Check sheet for the modelled part. Datum: model origin and axes. Units: mm. A direction names the side the tool comes from. Coordinates: 2 decimals unless noted, no trailing zeros. Loops run counter-clockwise (first coordinate to the right, second up) from the corner with the lowest first, then second, coordinate; pieces in that order, holes last. Notation, with made-up numbers: (64, 70.5) -> (97, 70.5) arc R27 ccw to (97, 102.5) -> close; hole circle Ø6 at (88, 87.5). An arc over 180 degrees is marked (long way). Use CSV: the item, a comma, the result in double quotes. Start each with the question number.
1. Sectioned sample at B-B, the plane x = 4. Record the cut outline in (y, z).
2. Set-up check for faces 1 (the face through (5, 6, 9)), 2 (the face through (5, 27.395, 10)), 3 (the face through (5, 14.942, 55)), 4 (the face through (5, -6.058, 56)): record each of +Z, -Z, +X, -X, +Y, -Y from which the full face is reachable in a straight line by a thin tool's end or side.
3. Sectioned sample at D-D, the plane z = 53.5. Record the cut outline in (x, y).
4. Thickness scan on L1, parallel to Z at x = 7.75, y = 19; L2, parallel to Y at x = 4.25, z = 61; L3, parallel to Z at x = 8, y = 9. Record the ranges inside material, lowest first.
5. Release check for a two-part mould opening along Y. For faces 5 (the face through (8, 12.395, 9)), 6 (the face through (5, 21, 24)), 7 (the face through (5, -16.003, 11)) record: pulls with the +Y half, pulls with the -Y half, needs draft (parallel to the pull), parting line crosses it, or undercut.
6. Sectioned sample at C-C, the plane y = 8.5. Record the cut outline in (x, z), and give its area (3 significant figures).
7. Sectioned sample at A-A, the plane z = 6. Record the cut outline in (x, y).
8. Gauge pin test, flat ends, axial feed: pin 1 (4 mm diameter, centred on x = 8.5, y = 8.5, fed in from -Z); pin 2 (2 mm diameter, centred on x = 3.5, y = -11.5, fed in from +Z); pin 3 (5 mm diameter, centred on x = 4.5, y = -6.5, fed in from +Z). Record the tip position at first contact, or that the pin passes through.
```python
from build123d import *

# Parameters (mm, degrees)
SALIENTE_EXTRUIR1_DEPTH = 10
CROQUIS2_W              = 18
CROQUIS2_H              = 12.394708995
CORTAR_EXTRUIR1_DEPTH   = 5
REDONDEO1_R             = 3
REDONDEO2_R             = 3
REDONDEO3_R             = 1


with BuildPart() as part:
    # Croquis1 → Saliente-Extruir1 (new body)
    with BuildSketch(Plane(origin=(0, 0, 0), x_dir=(0, 0, -1), z_dir=(1, 0, 0))):
        Polygon((0, -10.216508635), (0, 27.394708995), (-24, 27.394708995), (-24, 14.942424084), (-87.663818946, 14.942424084), (-87.663818946, -6.057575916), (-24, -6.057575916), (-24, -16.002849809), (0, -16.002849809), align=None)
    extrude(amount=SALIENTE_EXTRUIR1_DEPTH)

    # Croquis2 → Cortar-Extruir1 (cut)
    with BuildSketch(Plane(origin=(10, 0, 0), x_dir=(0, 0, -1), z_dir=(1, 0, 0))):
        with Locations((-9, 6.197354498)):
            Rectangle(CROQUIS2_W, CROQUIS2_H)
    extrude(amount=-CORTAR_EXTRUIR1_DEPTH, mode=Mode.SUBTRACT)

    # Redondeo1
    redondeo1_edges = [part.edges().sort_by_distance(p)[0] for p in [
        (5, -6.057575916, 24),
        (5, 14.942424084, 24),
    ]]
    fillet(redondeo1_edges, radius=REDONDEO1_R)

    # Redondeo2
    redondeo2_edges = [part.edges().sort_by_distance(p)[0] for p in [
        (5, -16.002849809, 24),
        (5, -6.057575916, 87.663818946),
        (5, 14.942424084, 87.663818946),
        (5, 27.394708995, 24),
    ]]
    fillet(redondeo2_edges, radius=REDONDEO2_R)

    # Redondeo3
    redondeo3_edges = [part.edges().sort_by_distance(p)[0] for p in [
        (7.5, 0, 18),
        (7.5, 12.394708995, 18),
    ]]
    fillet(redondeo3_edges, radius=REDONDEO3_R)


solid = part.part
```
Completed:
1,outline,"(-16, 0) -> (27.39, 0) -> (27.39, 21) arc R3 ccw to (24.39, 24) -> (17.94, 24) arc R3 cw to (14.94, 27) -> (14.94, 84.66) arc R3 ccw to (11.94, 87.66) -> (-3.06, 87.66) arc R3 ccw to (-6.06, 84.66) -> (-6.06, 27) arc R3 cw to (-9.06, 24) -> (-13, 24) arc R3 ccw to (-16, 21) -> close"
2,face 1,"-Z, +X"
2,face 2,"+Z, -Z, +X, -X, +Y"
2,face 3,"+Z, +X, -X, +Y"
2,face 4,"+Z, +X, -X, -Y"
3,outline,"(0, -6.06) -> (10, -6.06) -> (10, 14.94) -> (0, 14.94) -> close"
4,L1,"0 to 24"
4,L2,"-6.06 to 14.94"
4,L3,"18 to 87.66"
5,face 5,"undercut"
5,face 6,"needs draft"
5,face 7,"pulls with the -Y half"
6,outline,"(0, 0) -> (5, 0) -> (5, 18) -> (10, 18) -> (10, 87.66) -> (0, 87.66) -> close"
6,area,"787 mm²"
7,outline,"(0, -16) -> (10, -16) -> (10, 0) -> (5, 0) -> (5, 12.39) -> (10, 12.39) -> (10, 27.39) -> (0, 27.39) -> close"
8,pin 1,"z = 18"
8,pin 2,"z = 24"
8,pin 3,"z = 87.51"
